Source: CAD feature listing. Evaluate the final solid. Frame: model axes, mm. A direction names the side the tool comes from. Round coordinates to 2 decimals unless told otherwise and drop trailing zeros. Loops run counter-clockwise (first coordinate to the right, second up) from the corner with the lowest first, then second, coordinate; pieces in that order, holes last. Notation, with made-up numbers: (-17.75, -21.75) -> (-3.75, -21.75) arc R22 cw to (-3.75, 7.25) -> close; hole circle Ø6 at (-2, 8.5). An arc over 180 degrees is marked (long way). Write item = value, one per line.
from build123d import *

# Parameters (mm, degrees)
SKETCH1_W                = 64.3
SKETCH1_H                = 40.5
SKETCH1_R                = 1.5
BOSS_EXTRUDE1_DEPTH      = 2
SKETCH1_3_W              = 68.3
SKETCH1_3_H              = 44.5
SKETCH1_3_W_2            = 64.3
SKETCH1_3_H_2            = 40.5
BOSS_EXTRUDE2_DEPTH      = 4
BOSS_EXTRUDE3_DEPTH      = 32
BOSS_EXTRUDE3_DEPTH_BACK = 4
SKETCH5_R                = 2
BOSS_EXTRUDE4_DEPTH      = 3


with BuildPart() as part:
    # Sketch1 → Boss-Extrude1 (new body)
    with BuildSketch(Plane(origin=(0, 0, 0), x_dir=(1, 0, 0), z_dir=(0, 1, 0))):
        with Locations((2.688909091, -7.273090909)):
            Rectangle(SKETCH1_W, SKETCH1_H)
        with Locations(Location((-27.461090909, 8.976909091, 0), (0, 0, 270))):
            Circle(SKETCH1_R, mode=Mode.SUBTRACT)
        with Locations(Location((32.838909091, -23.523090909, 0), (0, 0, 270))):
            Circle(SKETCH1_R, mode=Mode.SUBTRACT)
        with Locations(Location((31.838909091, 10.476909091, 0), (0, 0, 270))):
            Circle(SKETCH1_R, mode=Mode.SUBTRACT)
        with Locations(Location((-26.461090909, -11.523090909, 0), (0, 0, 270))):
            Circle(SKETCH1_R, mode=Mode.SUBTRACT)
    extrude(amount=BOSS_EXTRUDE1_DEPTH)

    # Sketch1_3 → Boss-Extrude2 (add)
    with BuildSketch(Plane(origin=(0, 0, 0), x_dir=(1, 0, 0), z_dir=(0, 1, 0))):
        with Locations((2.688909091, -7.273090909)):
            Rectangle(SKETCH1_3_W, SKETCH1_3_H)
        with Locations((2.688909091, -7.273090909)):
            Rectangle(SKETCH1_3_W_2, SKETCH1_3_H_2, mode=Mode.SUBTRACT)
    extrude(amount=BOSS_EXTRUDE2_DEPTH)

    # Sketch3 → Boss-Extrude3 (add, two sides: drawn at the far end of the back side and taken through both)
    with BuildSketch(Plane.XZ.offset(-BOSS_EXTRUDE3_DEPTH_BACK)):
        Polygon((-31.461090909, -14.976909091), (36.838909091, -14.976909091), (36.838909091, -12.977521958), (-29.461090909, -12.977521958), (-29.461090909, 27.446996909), (36.838909091, 27.446996909), (36.838909091, 29.523090909), (-31.461090909, 29.523090909), align=None)
    extrude(amount=BOSS_EXTRUDE3_DEPTH + BOSS_EXTRUDE3_DEPTH_BACK)

    # Sketch5 → Boss-Extrude4 (add)
    # profile 1 of 2: a face of its own
    with BuildSketch(Plane.XZ.offset(32)):
        with BuildLine():
            Line((4.538909091, 29.523090909), (4.538909091, 35.523090909))
            ThreePointArc((4.538909091, 35.523090909), (-1.461090909, 41.523090909), (-7.461090909, 35.523090909))
            Line((-7.461090909, 35.523090909), (-7.461090909, 29.523090909))
            Line((-7.461090909, 29.523090909), (4.538909091, 29.523090909))
        make_face()
        with Locations(Location((-1.461090909, 35.523090909, 0), (0, 0, 270))):
            Circle(SKETCH5_R, mode=Mode.SUBTRACT)
    # profile 2 of 2: a face of its own
    with BuildSketch(Plane.XZ.offset(32)):
        with BuildLine():
            Line((4.538909091, -14.976909091), (-7.461090909, -14.976909091))
            Line((-7.461090909, -14.976909091), (-7.461090909, -21.053615958))
            ThreePointArc((-7.461090909, -21.053615958), (-1.461090909, -27.053615958), (4.538909091, -21.053615958))
            Line((4.538909091, -21.053615958), (4.538909091, -14.976909091))
        make_face()
        with Locations(Location((-1.461090909, -21.053615958, 0), (0, 0, 270))):
            Circle(SKETCH5_R, mode=Mode.SUBTRACT)
    extrude(amount=-BOSS_EXTRUDE4_DEPTH)


solid = part.part
1. Section query C-C (z = -20). Return the cut outline in (x, y).
Evaluation:
outline = (-7.46, -32) -> (-3.16, -32) -> (-3.16, -29) -> (-7.46, -29) -> close; (0.24, -32) -> (4.54, -32) -> (4.54, -29) -> (0.24, -29) -> close
2. Section query D-D (x = 16.5). Return the cut outline in (y, z), then the cut area to 3 significant figures.
Evaluation:
outline = (-32, -14.98) -> (4, -14.98) -> (4, -12.98) -> (2, -12.98) -> (2, 27.45) -> (4, 27.45) -> (4, 29.52) -> (-32, 29.52) -> (-32, 27.45) -> (0, 27.45) -> (0, -12.98) -> (-32, -12.98) -> close
area = 228 mm²
3. Section query A-A (z = -2). Return the cut outline in (x, y).
Evaluation:
outline = (-31.46, -32) -> (-29.46, -32) -> (-29.46, 0) -> (36.84, 0) -> (36.84, 4) -> (34.84, 4) -> (34.84, 2) -> (-29.46, 2) -> (-29.46, 4) -> (-31.46, 4) -> close
4. Mould query, pull axis Z, two halves, no side actions, for faces 1 (the face through (-7.461, -31, 33)), 2 (the face through (-1.593, -30.521, -27.052)), 3 (the face through (4, -16, -12.978)), 4 (the face through (34.839, 3, 8)). Classes: released by +Z, released by -Z, zero draft, split by the parting line, or undercut.
Evaluation:
face_1 = zero draft
face_2 = released by -Z
face_3 = undercut
face_4 = undercut
5. Line query: probe 1 along Z at (x, y) = (14, -20); probe 2 along X at (y, z) = (1, 23.5); probe 3 along Y at (x, z) = (31, 25). Output: solid intervals per line, ascending. Write a range as from..to.
Evaluation:
probe_1 = -14.98..-12.98, 27.45..29.52
probe_2 = -31.46..31.34, 34.34..36.84
probe_3 = 0..2
6. Section query B-B (y = -7.5). Return the cut outline in (x, z), then the cut area to 3 significant figures.
Evaluation:
outline = (-31.46, -14.98) -> (36.84, -14.98) -> (36.84, -12.98) -> (-29.46, -12.98) -> (-29.46, 27.45) -> (36.84, 27.45) -> (36.84, 29.52) -> (-31.46, 29.52) -> close
area = 359 mm²
7. Set-up query: faces 5 (the face through (36.839, 1, 7)), 6 (the face through (-2, -29, -18)), 7 (the face through (30.375, 0.986, -10.802)), 8 (the face through (-29.461, -16, 7)), 9 (the face through (2, 3, 27.447)). Return all of +Z, -Z, +X, -X, +Y, -Y with unobstructed straight access to the full face (end or side cutting, diameter ignored); none if empty.
Evaluation:
face_5 = +Z, -Z, +X, +Y, -Y
face_6 = -Z, +X, -X, +Y
face_7 = +Y, -Y
face_8 = +X, -Y
face_9 = +Y
8. Contact query for flat-ended pins moving along their axis: pin 1 Ø1.5 at (x, y) = (20.5, -1) entering from -Z; pin 2 Ø1.5 at (x, z) = (-14, 24.5) entering from -Y; pin 3 Ø5 at (x, z) = (-27.46, -8.98) entering from +Y; pin 4 Ø10 at (x, z) = (-13.5, -0.5) entering from +Y. Output: stop coordinate, or through.
Evaluation:
pin_1 = -14.98
pin_2 = 0
pin_3 = 4
pin_4 = 2
